For this review, take the finished solid that the model builds, in its own axes (mm). Face numbers are marked on the shaded views. A direction names the side the tool comes from. Round coordinates to 2 decimals unless told otherwise and drop trailing zeros. Loops run counter-clockwise (first coordinate to the right, second up) from the corner with the lowest first, then second, coordinate; pieces in that order, holes last.
1. Draft analysis for pull direction Z (two halves, no side actions). For the marked faces 1, 2, 3 and 4, state which applies: released by +Z, released by -Z, zero draft, split by the parting line, or undercut.
2. Clearance check with flat-ended pins moving along their axes: pin 1 Ø2.5 at (y, z) = (-32.5, -11) entering from -X; pin 2 Ø2.5 at (y, z) = (-30, -14.5) entering from +X; pin 3 Ø4 at (y, z) = (-29, -21) entering from -X. State where each tip first meets the part, or that it passes through.
3. Tool access review of the marked faces 5 and 6: name each direction out of +Z, -Z, +X, -X, +Y, -Y from which nothing blocks a thin tool from reaching the whole face with its end or side.
4. Consider section A-A on x = -3.75. State the section outline as (y, z) points, then the cut area to 3 significant figures.
5. Consider section B-B on x = 0.25. State the section outline as (y, z) points, then the cut area to 3 significant figures.
6. Consider section C-C on x = 4. State the section outline as (y, z) points, then the cut area to 3 significant figures.
7. To check wall thickness, follow line 1 along X through (y, z) = (-22, -15.25); line 2 along X through (y, z) = (-26.75, -3.5); line 3 along Y through (x, z) = (3.5, -5). State the ranges of each line that lie inside material, in increasing order.
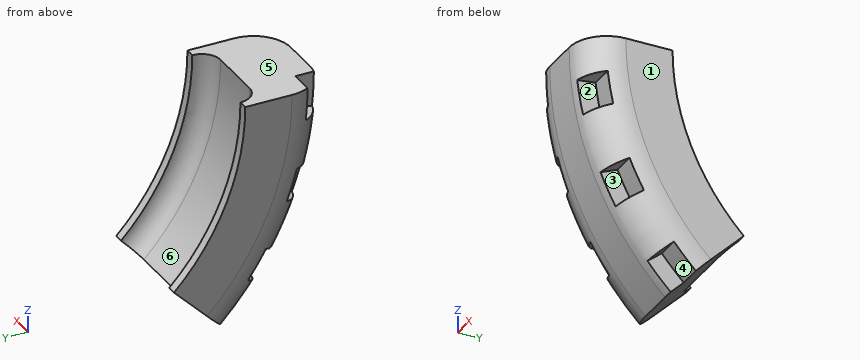
from build123d import *

# Parameters (mm, degrees)
REVOLVE1_ANGLE     = 45
CUT_EXTRUDE1_START = -3
CUT_EXTRUDE1_DEPTH = 3
CUT_EXTRUDE2_DEPTH = 3
FILLET1_R          = 2


with BuildPart() as part:
    # Sketch1 → Revolve1 (revolve)
    with BuildSketch(Plane.XY):
        with BuildLine():
            Line((-5, -28), (5, -28))
            Line((5, -28), (5, -26))
            Line((5, -26), (6, -26))
            Line((6, -26), (6, -31))
            ThreePointArc((6, -31), (4.828427125, -33.828427125), (2, -35))
            Line((2, -35), (-2, -35))
            ThreePointArc((-2, -35), (-4.828427125, -33.828427125), (-6, -31))
            Line((-6, -31), (-6, -26))
            Line((-6, -26), (-5, -26))
            Line((-5, -26), (-5, -28))
        make_face()
    revolve(axis=Axis((0.352941176, 0, 0), (1, 0, 0)), revolution_arc=REVOLVE1_ANGLE)

    # Sketch2 → Cut-Extrude1 (cut)
    with BuildSketch(Plane(origin=(6, 0, 0), x_dir=(0, 0, -1), z_dir=(1, 0, 0)).offset(CUT_EXTRUDE1_START)):
        with BuildLine():
            Line((21.979575266, -27.237809588), (20.66080075, -25.603541012))
            ThreePointArc((20.66080075, -25.603541012), (21.993442367, -24.468316101), (23.263813101, -23.263813101))
            Line((23.263813101, -23.263813101), (24.748737342, -24.748737342))
            ThreePointArc((24.748737342, -24.748737342), (23.397279114, -26.030123512), (21.979575266, -27.237809588))
        make_face()
        with BuildLine():
            Line((15.87243062, -28.817979565), (16.88556449, -30.657425069))
            ThreePointArc((16.88556449, -30.657425069), (15.230946014, -31.512192617), (13.533203573, -32.277738475))
            Line((13.533203573, -32.277738475), (12.721211358, -30.341074166))
            ThreePointArc((12.721211358, -30.341074166), (14.317089253, -29.62146106), (15.87243062, -28.817979565))
        make_face()
        with BuildLine():
            Line((7.227552694, -32.09630013), (7.688885845, -34.145000139))
            ThreePointArc((7.688885845, -34.145000139), (5.861777513, -34.505645399), (4.018072504, -34.768593491))
            Line((4.018072504, -34.768593491), (3.776988154, -32.682477882))
            ThreePointArc((3.776988154, -32.682477882), (5.510070862, -32.435306675), (7.227552694, -32.09630013))
        make_face()
    extrude(amount=CUT_EXTRUDE1_DEPTH, mode=Mode.SUBTRACT)

    # Sketch3 → Cut-Extrude2 (cut)
    with BuildSketch(Plane.ZY.offset(6)):
        with BuildLine():
            Line((0, -35), (0, -32.9))
            ThreePointArc((0, -32.9), (-1.752488008, -32.853291856), (-3.5, -32.713300048))
            Line((-3.5, -32.713300048), (-3.723404255, -34.801383029))
            ThreePointArc((-3.723404255, -34.801383029), (-1.864348945, -34.950310485), (0, -35))
        make_face()
        with BuildLine():
            Line((-12.636083101, -32.639384245), (-11.877918115, -30.68102119))
            ThreePointArc((-11.877918115, -30.68102119), (-10.226765616, -31.270165734), (-8.54657523, -31.770521743))
            Line((-8.54657523, -31.770521743), (-9.092101309, -33.798427386))
            ThreePointArc((-9.092101309, -33.798427386), (-10.879537889, -33.26613376), (-12.636083101, -32.639384245))
        make_face()
        with BuildLine():
            Line((-20.681152153, -28.236323161), (-19.440283023, -26.542143771))
            ThreePointArc((-19.440283023, -26.542143771), (-17.998860282, -27.539989625), (-16.506331561, -28.45963841))
            Line((-16.506331561, -28.45963841), (-17.559927193, -30.276211074))
            ThreePointArc((-17.559927193, -30.276211074), (-19.147723704, -29.297861303), (-20.681152153, -28.236323161))
        make_face()
    extrude(amount=-CUT_EXTRUDE2_DEPTH, mode=Mode.SUBTRACT)

    # Fillet1
    fillet1_edges = [part.edges().sort_by_distance(p)[0] for p in [
        (5, -25.86862691, -10.715136106),
        (-5, -25.86862691, -10.715136106),
    ]]
    fillet(fillet1_edges, radius=FILLET1_R - 0.0001)  # a hair under: the kernel refuses the full size


solid = part.part
Resolved:
1. face 1: zero draft
1. face 2: undercut
1. face 3: undercut
1. face 4: released by -Z
2. pin 1: stops at x = -3
2. pin 2: stops at x = 5.85
2. pin 3: stops at x = -4.84
3. face 5: +Z, +X, -X, +Y, -Y
3. face 6: +Z, +Y
4. outline: (-34.4, -3.68) arc R34.6 ccw to (-33.41, -8.99) - (-31.77, -8.55) arc R32.9 ccw to (-30.68, -11.88) - (-32.26, -12.49) arc R34.6 ccw to (-29.93, -17.36) - (-28.46, -16.51) arc R32.9 ccw to (-26.54, -19.44) - (-27.91, -20.44) arc R34.6 ccw to (-24.46, -24.46) - (-19.7, -19.7) arc R27.85 cw to (-27.85, 0) - (-32.9, 0) arc R32.9 ccw to (-32.71, -3.5) - close
4. area: 147 mm2
5. outline: (-35, 0) arc R35 ccw to (-24.75, -24.75) - (-19.8, -19.8) arc R28 cw to (-28, 0) - close
5. area: 173 mm2
6. outline: (-34.46, 0) arc R34.46 ccw to (-34.24, -3.96) - (-32.68, -3.78) arc R32.9 ccw to (-32.1, -7.23) - (-33.62, -7.57) arc R34.46 ccw to (-31.78, -13.33) - (-30.34, -12.72) arc R32.9 ccw to (-28.82, -15.87) - (-30.19, -16.63) arc R34.46 ccw to (-26.82, -21.64) - (-25.6, -20.66) arc R32.9 ccw to (-23.26, -23.26) - (-19.61, -19.61) arc R27.73 cw to (-27.73, 0) - close
6. area: 148 mm2
7. line 1: x = -6 to -4.85, 4.85 to 6
7. line 2: x = -6 to -4.74, 4.74 to 6
7. line 3: y = -32.52 to -27.49
